Read the model definition and answer for the solid it produces. Units are mm, in the model's axes. A direction names the side the tool comes from. Round coordinates to 2 decimals unless told otherwise and drop trailing zeros. Write each loop counter-clockwise with the first axis right and the second up, starting at its lowest first coordinate (ties: lowest second). Pieces come first, ordered by that corner, then holes.
Autodesk Inventor part; units mm, degrees
ref_plane "YZ Plane" through (0, 0, 0) normal (1, 0, 0) x (0, 1, 0)
ref_plane "XZ Plane" through (0, 0, 0) normal (0, 1, 0) x (-1, 0, 0)
ref_plane "XY Plane" through (0, 0, 0) normal (0, 0, 1) x (1, 0, 0)
sketch "Sketch1" plane through (0, 0, 0) normal (0, 0, 1) x (1, 0, 0)
  line L0 (0, 0) -> (20, 0)
  line L1 (20, 0) -> (20, 80)
  line L2 (20, 80) -> (0, 80)
  line L3 (0, 80) -> (0, 0)
  circle A0 centre (10, 70) radius 5.5
  line L4 (20, 0) -> (0, 0)
  line L5 (0, 0) -> (0, 3)
  line L6 (0, 3) -> (20, 3)
  line L7 (20, 3) -> (20, 0)
  point P0 (10, 0)
  dimension "d0" = 20
  dimension "d1" = 80
  dimension "d2" = 11
  dimension "d3" = 70
  dimension "d7" = 3
extrude "Extrusion1" add sketch "Sketch1" along normal blind 3
fillet "Fillet1" radius 5 2 edges at (20, 80, 1.5) (0, 80, 1.5)
extrude "Extrusion2" add sketch "Sketch1" against normal blind 30 contours L3 L6 L1 L0
sketch "Sketch2" plane through (0, 3, 0) normal (0, 1, 0) x (1, 0, 0)
  circle A0 centre (10, 22.1006) radius 2.5
  circle A1 centre (10, 10.048) radius 2.5
  point P0 (0, 0)
  dimension "d10" = 5
  dimension "d11" = 5
extrude "Extrusion3" cut sketch "Sketch2" against normal through all
extrude "Extrusion4" cut sketch "Sketch1" along normal blind 10 contours A0
extrude "Extrusion5" cut sketch "Sketch1" along normal blind 10 contours A0
sketch "Sketch3" plane through (0, 0, 3) normal (0, 0, 1) x (1, 0, 0)
  circle A0 centre (10, 53.969) radius 2.5
  circle A1 centre (10, 70) radius 5.5
  circle A2 centre (14.5, 53.969) radius 2.25
  circle A3 centre (5.5, 53.969) radius 2.25
  point P0 (0, 0)
  point P1 (7.6181, 54.7282)
  point P2 (7.6181, 53.2098)
  point P3 (12.3819, 53.2098)
  point P4 (12.3819, 54.7282)
  dimension "d18" = 5
  dimension "d19" = 16.031
  dimension "d20" = 4.5
  dimension "d21" = 4.5
  dimension "d22" = 4.5
  dimension "d23" = 4.5
extrude "Extrusion6" cut sketch "Sketch3" against normal blind 1 contours A0 A2 | A0 A2 | A2 A0 A3 | A3 A0 | A0 A3
extrude "Extrusion7" cut sketch "Sketch3" against normal through all contours A0 A2 | A2 A0 A3 | A3 A0 picked at (12.3432, 53.969) picked at (7.5921, 53.969)
sketch "Sketch4" plane through (0, 0, 2) normal (0, 0, 1) x (1, 0, 0)
  arc A0 (7.6181, 54.7282) -> (7.6181, 53.2098) centre (5.5, 53.969) ccw
  circle A1 centre (5.5, 53.969) radius 1.25
  arc A2 (12.3819, 53.2098) -> (12.3819, 54.7282) centre (14.5, 53.969) ccw
  circle A3 centre (14.5, 53.969) radius 1.25
  point P0 (0, 0)
  dimension "d28" = 2.5
  dimension "d29" = 2.5
extrude "Extrusion8" cut sketch "Sketch4" against normal through all
properties part number "roll stand 1"
Q1. Flat-ended cylindrical pins translate along their axes: pin 1 Ø6.5 at (x, y) = (10, 53.969) entering from -Z; pin 2 Ø8 at (x, z) = (13, -20) entering from +Y; pin 3 Ø10 at (x, z) = (16.5, -17.5) entering from -Y; pin 4 Ø2 at (x, y) = (6.5, 53.5) entering from +Z. Find the tip coordinate at first contact, or state that the pin passes through.
Verdict:
pin 1: stops at z = 0
pin 2: stops at y = 3
pin 3: stops at y = 0
pin 4: stops at z = 2
Q2. Straight lines are drawn through the part: probe 1 along Z at (x, y) = (10, 2.25); probe 2 along Y at (x, z) = (5.5, 2.8); probe 3 along Y at (x, z) = (14.5, 0.45). For each, find the intervals that lie inside material, in ascending order.
Verdict:
probe 1: z = -30 to -24.6, -19.6 to -12.55, -7.55 to 3
probe 2: y = 0 to 51.72, 56.22 to 66.84, 73.16 to 80
probe 3: y = 0 to 52.72, 55.22 to 66.84, 73.16 to 80
Q3. Section D-D (x = 14) is taken. Determine the outline of the cut face in (y, z).
Verdict:
outline: (0, -30) - (3, -30) - (3, 0) - (52.82, 0) - (52.82, 2) - (51.78, 2) - (51.78, 3) - (0, 3) - close; (55.11, 0) - (66.23, 0) - (66.23, 3) - (56.16, 3) - (56.16, 2) - (55.11, 2) - close; (73.77, 0) - (80, 0) - (80, 3) - (73.77, 3) - close
Q4. Determine the mould class of faces 1 (the flat face through (16, 53, 2)), 2 (the cylindrical face through (9.284, 64.547, 1.479)), 3 (the cylindrical face through (9.5, 1.5, -7.6)) for opening direction Z: pulls with the +Z half, pulls with the -Z half, needs draft (parallel to the pull), parting line crosses it, or undercut.
Verdict:
face 1: pulls with the +Z half
face 2: needs draft
face 3: undercut
Q5. Section B-B (x = 10) is taken. Determine the outline of the cut face in (y, z).
Verdict:
outline: (0, -30) - (3, -30) - (3, -24.6) - (0, -24.6) - close; (0, -19.6) - (3, -19.6) - (3, -12.55) - (0, -12.55) - close; (0, -7.55) - (3, -7.55) - (3, 0) - (51.47, 0) - (51.47, 3) - (0, 3) - close; (56.47, 0) - (64.5, 0) - (64.5, 3) - (56.47, 3) - close; (75.5, 0) - (80, 0) - (80, 3) - (75.5, 3) - close
Q6. Section A-A (y = 70) is taken. Determine the outline of the cut face in (x, z).
Verdict:
outline: (0, 0) - (4.5, 0) - (4.5, 3) - (0, 3) - close; (15.5, 0) - (20, 0) - (20, 3) - (15.5, 3) - close
Q7. Which of the six approach directions +Z, -Z, +X, -X, +Y, -Y give full straight-line access (tool end or side, diameter ignored) to faces 4 (the flat face through (7, 54, 2)), 5 (the flat face through (10, 42, 0)), 6 (the flat face through (10, 80, 1))?
Verdict:
face 4: +Z
face 5: -Z, +X, -X, +Y
face 6: +Z, -Z, +X, -X, +Y
Q8. Section C-C (z = -21) is taken. Determine the outline of the cut face in (x, y).
Verdict:
outline: (0, 0) - (7.76, 0) - (7.76, 3) - (0, 3) - close; (12.24, 0) - (20, 0) - (20, 3) - (12.24, 3) - close
